```python
from build123d import *

# Parameters (mm, degrees)
SKETCH1_W           = 45
SKETCH1_H           = 20.5
BOSS_EXTRUDE2_DEPTH = 3.556
SKETCH2_R           = 7.9375
BOSS_EXTRUDE3_DEPTH = 12.7
SKETCH3_R           = 6.1595
CUT_EXTRUDE1_DEPTH  = 0.635
SKETCH4_W           = 10.16
SKETCH4_H           = 3.81
BOSS_EXTRUDE4_DEPTH = 3.302
FILLET1_R           = 1.27
FILLET2_R           = 0.254
SKETCH5_R           = 0.762
CUT_EXTRUDE2_DEPTH  = 3.302


with BuildPart() as part:
    # Sketch1 → Boss-Extrude2 (new body)
    with BuildSketch(Plane.XY):
        Rectangle(SKETCH1_W, SKETCH1_H)
    extrude(amount=BOSS_EXTRUDE2_DEPTH)

    # Sketch2 → Boss-Extrude3 (add)
    with BuildSketch(Plane.XY.offset(3.556)):
        with Locations(Location((13.2, 0, 0), (0, 0, 180))):
            Circle(SKETCH2_R)
        with Locations(Location((-13.2, 0, 0), (0, 0, 180))):
            Circle(SKETCH2_R)
    extrude(amount=BOSS_EXTRUDE3_DEPTH)

    # Sketch3 → Cut-Extrude1 (cut)
    with BuildSketch(Plane.XY.offset(16.256)):
        with Locations((-13.2, 0)):
            Circle(SKETCH3_R)
        with Locations(Location((13.2, 0, 0), (0, 0, 180))):
            Circle(SKETCH3_R)
    extrude(amount=-CUT_EXTRUDE1_DEPTH, mode=Mode.SUBTRACT)

    # Sketch4 → Boss-Extrude4 (add)
    with BuildSketch(Plane.XY.offset(3.556)):
        with Locations((0, 7.71)):
            Rectangle(SKETCH4_W, SKETCH4_H)
    extrude(amount=BOSS_EXTRUDE4_DEPTH)

    # Fillet1
    fillet1_edges = [part.edges().sort_by_distance(p)[0] for p in [
        (5.08, 5.805, 5.207),
        (5.08, 9.615, 5.207),
        (-5.08, 9.615, 5.207),
        (-5.08, 5.805, 5.207),
    ]]
    fillet(fillet1_edges, radius=FILLET1_R)

    # Fillet2
    fillet2_edges = [part.edges().sort_by_distance(p)[0] for p in [
        (21.1375, 0, 16.256),
        (-5.2625, 0, 16.256),
        (-19.3595, 0, 16.256),
        (19.3595, 0, 16.256),
        (5.08, 7.71, 6.858),
        (0, 5.805, 6.858),
        (0, 9.615, 6.858),
        (-5.08, 7.71, 6.858),
        (-4.708025612, 6.176974388, 6.858),
        (4.708025612, 9.243025612, 6.858),
        (-4.708025612, 9.243025612, 6.858),
        (4.708025612, 6.176974388, 6.858),
    ]]
    fillet(fillet2_edges, radius=FILLET2_R)

    # Sketch5 → Cut-Extrude2 (cut)
    with BuildSketch(Plane.XY.offset(3.556)):
        with Locations((21.484, -9.234)):
            Circle(SKETCH5_R)
        with Locations((21.484, 9.234)):
            Circle(SKETCH5_R)
        with Locations((-21.484, 9.234)):
            Circle(SKETCH5_R)
        with Locations((-21.484, -9.234)):
            Circle(SKETCH5_R)
    extrude(amount=-CUT_EXTRUDE2_DEPTH, mode=Mode.SUBTRACT)


solid = part.part
```
Build history of the part. All positions in model axes, mm. A direction names the side the tool comes from. Round coordinates to 2 decimals unless told otherwise and drop trailing zeros. Loops run counter-clockwise (first coordinate to the right, second up) from the corner with the lowest first, then second, coordinate; pieces in that order, holes last.
Item 1: Drill centre lines: line 1 along Y through (x, z) = (-13.2, 15.95); line 2 along X through (y, z) = (-2, 12); line 3 along Z through (x, y) = (-8.5, -7). Where is each one in solid material? Low to high.
Item 2: Saw through at B-B (x = 13.2). List the corners of the cut face in (y, z), then the cut area to 3 significant figures.
Item 3: Saw through at A-A (y = 0). List the corners of the cut face in (x, z), then the cut area to 3 significant figures.
Item 4: Pin check, flat tips, straight feed: P1, Ø1, axis at y = -2.5, z = 9, coming from the +X side; P2, Ø2.5, axis at x = 21.484, y = -9.234, coming from the +Z side; P3, Ø6, axis at x = 14, y = 0.5, coming from the +Z side. Stop position of each tip, or through.
Item 5: Two-plate mould, pull along Y, no slides. Class faces 1 (the face through (-20.771, -2.384, 9.692)), 2 (the face through (-22.09, 8.77, 1.93)), 3 (the face through (0, 8, 6.858)): released by +Y, released by -Y, zero draft, split by the parting line, or undercut.
Item 6: Which spindle directions (+Z, -Z, +X, -X, +Y, -Y) get a long thin tool onto all of the face, cutting with end or side? Do faces 4 (the face through (0, 9.615, 5)), 5 (the face through (-13, 0, 15.621)), 6 (the face through (-5.08, 8, 5)), 7 (the face through (-4.7, 9.25, 5.1)), 8 (the face through (4.7, 6.17, 5.1)). Say none if no direction does.
Item 7: Saw through at C-C (z = 9). List the corners of the cut face in (x, y) (1 decimal).
Worked answers:
1. line 1: y = -7.94 to -6.16, 6.16 to 7.94
1. line 2: x = -20.88 to -5.52, 5.52 to 20.88
1. line 3: z = 0 to 3.56
2. outline: (-10.25, 0) - (10.25, 0) - (10.25, 3.56) - (7.94, 3.56) - (7.94, 16) arc R0.25 ccw to (7.68, 16.26) - (6.41, 16.26) arc R0.25 ccw to (6.16, 16) - (6.16, 15.62) - (-6.16, 15.62) - (-6.16, 16) arc R0.25 ccw to (-6.41, 16.26) - (-7.68, 16.26) arc R0.25 ccw to (-7.94, 16) - (-7.94, 3.56) - (-10.25, 3.56) - close
2. area: 267 mm2
3. outline: (-22.5, 0) - (22.5, 0) - (22.5, 3.56) - (21.14, 3.56) - (21.14, 16) arc R0.25 ccw to (20.88, 16.26) - (19.61, 16.26) arc R0.25 ccw to (19.36, 16) - (19.36, 15.62) - (7.04, 15.62) - (7.04, 16) arc R0.25 ccw to (6.79, 16.26) - (5.52, 16.26) arc R0.25 ccw to (5.26, 16) - (5.26, 3.56) - (-5.26, 3.56) - (-5.26, 16) arc R0.25 ccw to (-5.52, 16.26) - (-6.79, 16.26) arc R0.25 ccw to (-7.04, 16) - (-7.04, 15.62) - (-19.36, 15.62) - (-19.36, 16) arc R0.25 ccw to (-19.61, 16.26) - (-20.88, 16.26) arc R0.25 ccw to (-21.14, 16) - (-21.14, 3.56) - (-22.5, 3.56) - close
3. area: 547 mm2
4. P1: stops at x = 20.88
4. P2: stops at z = 3.56
4. P3: stops at z = 15.62
5. face 1: split by the parting line
5. face 2: undercut
5. face 3: zero draft
6. face 4: +Z, +X, -X, +Y
6. face 5: +Z
6. face 6: +Z, +Y, -Y
6. face 7: +Z, -X, +Y
6. face 8: +Z, -Y
7. outline: circle Ø15.9 at (-13.2, 0); circle Ø15.9 at (13.2, 0)
